Work out the finished part from the listing and answer in its coordinate system (mm). Give positions to 0.01 mm unless a question says otherwise; leave off trailing zeros. Loops run counter-clockwise (first coordinate to the right, second up) from the corner with the lowest first, then second, coordinate; pieces in that order, holes last. Notation, with made-up numbers: (-25.5, 77) - (-5.5, 77) arc R13 cw to (-5.5, 91) - close; hole circle Ø4 at (0.25, 73.5). An arc over 180 degrees is marked (long way). One line per question, with ' | ' between items.
from build123d import *

# Parameters (mm, degrees)
F0_R     = 17.5
F0_R_2   = 13.5
F1_DEPTH = 5
F2_R     = 0.25
F3_R     = 16
F4_DEPTH = 2
F5_R     = 1.99999


# Not quite as in the source:
# - a fillet or chamfer is up to 0.001 mm smaller than in the source, because OpenCascade refuses the exact size


with BuildPart() as f1:
    # F0 (on Front) → F1 (new body)
    with BuildSketch(Plane.XZ):
        Circle(F0_R)
        Circle(F0_R_2, mode=Mode.SUBTRACT)
    extrude(amount=F1_DEPTH)

    # F2
    f2_edges = [f1.edges().sort_by_distance(p)[0] for p in [
        (-17.5, -5, 0),
        (-13.5, -5, 0),
    ]]
    fillet(f2_edges, radius=F2_R)

    # F3 (on Front) → F4 (cut)
    with BuildSketch(Plane.XZ):
        Circle(F3_R)
    extrude(amount=F4_DEPTH, mode=Mode.SUBTRACT)

    # F5 (radius 2 in the source; OpenCascade refuses exactly that, so slightly less here)
    f5_edges = [f1.edges().sort_by_distance(p)[0] for p in [
        (-16, -2, 0),
    ]]
    fillet(f5_edges, radius=F5_R)


solid = f1.part
1. Flat-ended cylindrical pins translate along their axes: pin 1 (1 mm diameter, centred on y = -2.5, z = -4, fed in from -X); pin 2 (5 mm diameter, centred on x = -5, z = 11.5, fed in from +Y); pin 3 (8.5 mm diameter, centred on x = -5.5, z = -4, fed in from +Y). Find the tip coordinate at first contact, or state that the pin passes through.
Evaluation:
pin 1: x = -17.15 | pin 2: y = -1.71 | pin 3: through
2. Consider L1, parallel to Z at x = 0, y = -3.55; L2, parallel to X at y = -1.6, z = 3.5; L3, parallel to Z at x = 4.5, y = -2.3. Determine where each line is inside the solid, lowest interval first.
Evaluation:
L1: -17.5 to -13.5, 13.5 to 17.5 | L2: -17.15 to -14.79, 14.79 to 17.15 | L3: -16.91 to -12.73, 12.73 to 16.91
3. Determine the mould class of faces 1 (the flat face through (-12, -5, -8)), 2 (the cylindrical face through (-2.93, -3.36, -13.18)), 3 (the cylindrical face through (-13.887, -2.342, -10.648)) for opening direction Z: +Z half, -Z half, draft (parallel to the pull), parting line (faces both ways), or undercut.
Evaluation:
face 1: draft | face 2: undercut | face 3: parting line
4. Find section C-C on y = -4.2. Write down the section's boundary in (x, z).
Evaluation:
outline: circle Ø35 at (0, 0); hole circle Ø27 at (0, 0)
